Check sheet for the modelled part. Datum: model origin and axes. Units: mm. A direction names the side the tool comes from. Round coordinates to 2 decimals unless told otherwise and drop trailing zeros. Order: outer loops, then holes, each group sorted by start corner. A loop starts at its lowest first (then second) coordinate and runs counter-clockwise, first axis right, second up.
```python
from build123d import *

# Parameters (mm, degrees)
EXTRUDE_1_DEPTH = 10
FILLET_1_R      = 5
FILLET_2_R      = 5


with BuildPart() as part:
    # 草图1 → 凸台-拉伸1 (new body)
    with BuildSketch(Plane(origin=(0, 0, 0), x_dir=(1, 0, 0), z_dir=(0, 1, 0))):
        Polygon((0, 0), (600, 0), (600, 200), (610, 200), (610, -10), (600, -10), (0, -10), align=None)
    extrude(amount=EXTRUDE_1_DEPTH)

    # 圆角1
    fillet_1_edges = [part.edges().sort_by_distance(p)[0] for p in [
        (600, 5, 0),
    ]]
    fillet(fillet_1_edges, radius=FILLET_1_R)

    # 圆角2
    fillet_2_edges = [part.edges().sort_by_distance(p)[0] for p in [
        (610, 5, 10),
    ]]
    fillet(fillet_2_edges, radius=FILLET_2_R)


solid = part.part
```
Item 1: Go/stop test with flat-tipped pins: P1, Ø2, axis at y = 8.5, z = -146.5, coming from the -X side; P2, Ø5, axis at x = 318.5, y = 5.5, coming from the -Z side. Record where each tip stops, or that it passes through.
Answer:
P1: stops at x = 600
P2: stops at z = 0
Item 2: Sectioned sample at B-B (z = -183.5). Record the cut outline in (x, y), and give its area (3 significant figures).
Answer:
outline: (600, 0) - (610, 0) - (610, 10) - (600, 10) - close
area: 100 mm2
Item 3: Scan lines: line 1 along X through (y, z) = (8.75, -120); line 2 along Z through (x, y) = (130, 7.5). Record each from-to range of solid material in increasing order.
Answer:
line 1: x = 600 to 610
line 2: z = 0 to 10
Item 4: Sectioned sample at A-A (y = 7.5). Record the cut outline in (x, z).
Answer:
outline: (0, 0) - (595, 0) arc R5 cw to (600, -5) - (600, -200) - (610, -200) - (610, 5) arc R5 ccw to (605, 10) - (0, 10) - close
Item 5: Sectioned sample at C-C (x = 105.5). Record the cut outline in (y, z), and give its area (3 significant figures).
Answer:
outline: (0, 0) - (10, 0) - (10, 10) - (0, 10) - close
area: 100 mm2
Item 6: Access from +Z, -Z, +X, -X, +Y, -Y to the whole of each face (thin tool, end or side, straight path). Record for faces 1 (the flat face through (600, 5, -101)), 2 (the flat face through (442, 0, 6)).
Answer:
face 1: -Z, -X, +Y, -Y
face 2: +Z, -Z, +X, -X, -Y
